Source: CAD feature listing. Evaluate the final solid. Frame: model axes, mm. A direction names the side the tool comes from. Coordinates: 2 decimals unless noted, no trailing zeros. Write each loop counter-clockwise with the first axis right and the second up, starting at its lowest first coordinate (ties: lowest second). Pieces come first, ordered by that corner, then holes. Notation, with made-up numbers: (63, -29) -> (114, -29) arc R29 cw to (114, 9) -> close; hole circle Ø2 at (-37, 1.25). An arc over 180 degrees is marked (long way). Write item = value, one per line.
from build123d import *

# Parameters (mm, degrees)
F1_DEPTH  = 12.75
F3_DEPTH  = 2.5
F5_DEPTH  = 6.5
F7_DEPTH  = 40.9
F10_DEPTH = 27.7
F11_R     = 6
F11_R_2   = 4.9
F12_DEPTH = 30


with BuildPart() as f1:
    # F0 (on Front) → F1 (new body, symmetric)
    with BuildSketch(Plane.XZ):
        with BuildLine():
            Line((0, 36), (0, 0))
            Line((0, 0), (52, 0))
            Line((52, 0), (80, 13))
            Line((80, 13), (120, 13))
            Line((120, 13), (146, 22))
            Line((146, 22), (162, 30))
            Line((162, 30), (166, 33))
            Line((166, 33), (166, 47))
            Line((166, 47), (164, 52))
            Line((164, 52), (146.7757606487, 53.4353532793))
            ThreePointArc((146.7757606487, 53.4353532793), (147.6907523587, 50.5301477084), (148, 47.5))
            ThreePointArc((148, 47.5), (147.4913767462, 43.6270166538), (146, 40.0166852265))
            Line((146, 40.0166852265), (146, 36))
            Line((146, 36), (142.6306801421, 36))
            ThreePointArc((142.6306801421, 36), (133, 32.5), (123.3693198579, 36))
            Line((123.3693198579, 36), (0, 36))
        make_face()
        with BuildLine():
            ThreePointArc((146, 40.0166852265), (144.4921869536, 37.8599979759), (142.6306801421, 36))
            Line((142.6306801421, 36), (146, 36))
            Line((146, 36), (146, 40.0166852265))
        make_face()
    extrude(amount=F1_DEPTH, both=True)

    # F2 (on Front) → F3 (cut, symmetric)
    with BuildSketch(Plane.XZ):
        with BuildLine():
            Line((123.3693198579, 36), (119.1526175759, 36))
            ThreePointArc((119.1526175759, 36), (120.0845966785, 34.9623623819), (121.0941191002, 34))
            ThreePointArc((121.0941191002, 34), (142.9238149728, 32.4827467097), (150.0871635222, 53.1594030398))
            Line((150.0871635222, 53.1594030398), (146.7757606487, 53.4353532793))
            ThreePointArc((146.7757606487, 53.4353532793), (141.9606533855, 35.4705905837), (123.3693198579, 36))
        make_face()
    extrude(amount=F3_DEPTH, both=True, mode=Mode.SUBTRACT)

    # F4 (on Front) → F5 (cut, symmetric)
    with BuildSketch(Plane.XZ):
        Polygon((119.1526175759, 36), (0, 36), (0, 34), (121.0941191002, 34), (129.1526175759, 34), (129.1526175759, 36), align=None)
    extrude(amount=F5_DEPTH, both=True, mode=Mode.SUBTRACT)

    # F6 (on face) → F7 (cut)
    with BuildSketch(Plane.XY.offset(34)):
        with BuildLine():
            ThreePointArc((147.5, -6.5), (152.0961940777, -4.5961940777), (154, 0))
            ThreePointArc((154, 0), (152.0961940777, 4.5961940777), (147.5, 6.5))
            Line((147.5, 6.5), (147.5, -6.5))
        make_face()
        with BuildLine():
            Line((147.5, -6.5), (147.5, 6.5))
            ThreePointArc((147.5, 6.5), (141, 0), (147.5, -6.5))
        make_face()
        with BuildLine():
            ThreePointArc((147.5, -6.5), (141, 0), (147.5, 6.5))
            Line((147.5, 6.5), (132.5, 6.5))
            Line((132.5, 6.5), (132.5, -6.5))
            Line((132.5, -6.5), (147.5, -6.5))
        make_face()
    extrude(amount=F7_DEPTH, mode=Mode.SUBTRACT)

    # F9 (on offset) → F10 (cut)
    with BuildSketch(Plane.XY.offset(46)):
        with BuildLine():
            ThreePointArc((154.5, -6.5), (159.0961940777, -4.5961940777), (161, 0))
            ThreePointArc((161, 0), (159.0961940777, 4.5961940777), (154.5, 6.5))
            Line((154.5, 6.5), (154.5, -6.5))
        make_face()
        with BuildLine():
            Line((154.5, -6.5), (154.5, 6.5))
            ThreePointArc((154.5, 6.5), (148, 0), (154.5, -6.5))
        make_face()
        with BuildLine():
            ThreePointArc((154.5, -6.5), (148, 0), (154.5, 6.5))
            Line((154.5, 6.5), (139.5, 6.5))
            Line((139.5, 6.5), (139.5, -6.5))
            Line((139.5, -6.5), (154.5, -6.5))
        make_face()
    extrude(amount=F10_DEPTH, mode=Mode.SUBTRACT)

    # F11 (on face) → F12 (cut)
    with BuildSketch(Plane(origin=(0, 0, 0), x_dir=(0, -1, 0), z_dir=(-1, 0, 0))):
        with Locations((0, 21.2)):
            Circle(F11_R)
        with Locations((0, 21.2)):
            Circle(F11_R_2, mode=Mode.SUBTRACT)
        with Locations((0, 21.2)):
            Circle(F11_R_2)
    extrude(amount=-F12_DEPTH, mode=Mode.SUBTRACT)


solid = f1.part
1) Cut plane D-D, the plane z = 38. Output: boundary loops of the cut face in (x, y).
Answer block:
outline = (144.61, -12.75) -> (166, -12.75) -> (166, 12.75) -> (144.61, 12.75) -> (144.61, 6.5) -> (147.5, 6.5) arc R6.5 cw to (147.5, -6.5) -> (144.61, -6.5) -> close
2) First-contact query: pin 1 Ø3 at (x, y) = (73.5, 0.5) entering from -Z; pin 2 Ø12 at (y, z) = (5.5, 45.5) entering from -X; pin 3 Ø3 at (x, y) = (65, -10) entering from +Z. Flat tips, straight axial feed; report the tip coordinate or a pass-through.
Answer block:
pin_1 = 9.29
pin_2 = 145.74
pin_3 = 36
3) Cut plane C-C, the plane x = 111. Output: boundary loops of the cut face in (y, z), and give its area (4 significant figures).
Answer block:
outline = (-12.75, 13) -> (12.75, 13) -> (12.75, 36) -> (6.5, 36) -> (6.5, 34) -> (-6.5, 34) -> (-6.5, 36) -> (-12.75, 36) -> close
area = 560.5 mm2
4) Pull-direction query (Y, two-part tool) for faces 1 (the flat face through (65.804, -0.178, 6.409)), 2 (the flat face through (156, 0, 46)), 3 (the flat face through (82, 12.75, 21)); classes: +Y half, -Y half, draft (parallel to the pull), parting line (faces both ways), or undercut.
Answer block:
face_1 = draft
face_2 = undercut
face_3 = +Y half
5) Cut plane B-B, the plane y = -10.5. Output: boundary loops of the cut face in (x, z).
Answer block:
outline = (0, 0) -> (52, 0) -> (80, 13) -> (120, 13) -> (146, 22) -> (162, 30) -> (166, 33) -> (166, 47) -> (164, 52) -> (146.78, 53.44) arc R15 cw to (123.37, 36) -> (0, 36) -> close
6) Reachability of faces 4 (the flat face through (151, -6.5, 50)), 5 (the flat face through (133, 2.5, 32)), 6 (the flat face through (63, 10, 36)), 7 (the flat face through (161.25, -0.18, 52.23)), 8 (the cylindrical face through (14.79, 0.78, 27.15)) from +Z, -Z, +X, -X, +Y, -Y: full face, straight path, thin tool, end or side. Return the list, or none.
Answer block:
face_4 = +Z, -X
face_5 = +Z
face_6 = +Z, -X, +Y, -Y
face_7 = +Z, +X, +Y, -Y
face_8 = -X
7) Material intervals for probe 1 along Z at (x, y) = (21.75, 0); probe 2 along Z at (x, y) = (44, 5.5); probe 3 along Y at (x, z) = (24, 21), sorted ascending. Write a range as [from, to].
Answer block:
probe_1 = [0, 15.2], [27.2, 34]
probe_2 = [0, 34]
probe_3 = [-12.75, -6], [6, 12.75]
8) Cut plane A-A, the plane x = 17.5. Output: boundary loops of the cut face in (y, z), and give its area (3 significant figures).
Answer block:
outline = (-12.75, 0) -> (12.75, 0) -> (12.75, 36) -> (6.5, 36) -> (6.5, 34) -> (-6.5, 34) -> (-6.5, 36) -> (-12.75, 36) -> close; hole circle Ø12 at (0, 21.2)
area = 779 mm2
